Work out the finished part from the listing and answer in its coordinate system (mm). Face numbers are marked on the shaded views. A direction names the side the tool comes from. Coordinates: 2 decimals unless noted, no trailing zeros. Order: outer loops, then holes, each group sorted by start corner. A loop starts at its lowest first (then second) coordinate and runs counter-clockwise, first axis right, second up. Notation, with made-up numbers: (75, 31) - (129, 31) arc R10 ccw to (129, 43) - close; hole circle Ø8 at (31, 20.5). An arc over 180 degrees is marked (long way). Use CSV: the item, a comma, the result in double quotes. Start each with the question number.
from build123d import *

# Parameters (mm, degrees)
F0_W      = 18
F0_H      = 91.5
F0_W_2    = 7.2
F0_H_2    = 3.15
F0_W_3    = 12
F0_H_3    = 34
F1_DEPTH  = 10
F2_R      = 6
F4_DEPTH  = 7
F5_SIZE   = 2
F6_R      = 1.65
F7_DEPTH  = 25
F8_DEPTH  = 3
F10_R     = 4.99999
F12_DEPTH = 2.4
F15_DEPTH = 2.5
F17_R     = 2.15
F18_DEPTH = 20
F20_W     = 7.2
F20_H     = 3.15
F21_DEPTH = 1.25


# Not quite as in the source:
# - a fillet or chamfer is up to 0.001 mm smaller than in the source, because OpenCascade refuses the exact size


with BuildPart() as f1:
    # F0 (on Top) → F1 (new body)
    with BuildSketch(Plane.XY):
        with Locations((0.4665288143, 11.6095117688)):
            Rectangle(F0_W, F0_H)
        with Locations((0, -28.5654882312)):
            Rectangle(F0_W_2, F0_H_2, mode=Mode.SUBTRACT)
        Polygon((6.5, -24.9904882312), (-6.5, -24.9904882312), (-6.5, -15.9904882312), (0, -9.9904882312), (6.5, -15.9904882312), align=None, mode=Mode.SUBTRACT)
        with Locations((0.4665288143, 11.0095117688)):
            Rectangle(F0_W_3, F0_H_3, mode=Mode.SUBTRACT)
        with Locations((0.4665288143, 11.0095117688)):
            Rectangle(F0_W_3, F0_H_3)
    extrude(amount=F1_DEPTH)

    # F2
    f2_edges = [f1.edges().sort_by_distance(p)[0] for p in [
        (9.466529, -34.140488, 5),
        (-8.533471, -34.140488, 5),
    ]]
    fillet(f2_edges, radius=F2_R)

    # F0 (on Top) → F4 (cut)
    with BuildSketch(Plane.XY):
        with Locations((0.4665288143, 11.0095117688)):
            Rectangle(F0_W_3, F0_H_3)
    extrude(amount=F4_DEPTH, mode=Mode.SUBTRACT)

    # F5
    f5_edges = [f1.edges().sort_by_distance(p)[0] for p in [
        (6.466529, 11.009512, 7),
        (-5.533471, 11.009512, 7),
    ]]
    chamfer(f5_edges, length=F5_SIZE)

    # F6 (on offset) → F7 (cut)
    with BuildSketch(Plane.YZ.offset(9.4665288143)):
        with BuildLine():
            Line((40.3595117688, 3.35), (40.3595117688, 6.65))
            ThreePointArc((40.3595117688, 6.65), (38.7095117688, 5), (40.3595117688, 3.35))
        make_face()
        with BuildLine():
            ThreePointArc((42.0095117688, 5), (41.5262379578, 6.166726189), (40.3595117688, 6.65))
            Line((40.3595117688, 6.65), (40.3595117688, 3.35))
            ThreePointArc((40.3595117688, 3.35), (41.5262379578, 3.833273811), (42.0095117688, 5))
        make_face()
        with Locations((52.3595117688, 5)):
            Circle(F6_R)
    extrude(amount=-F7_DEPTH, mode=Mode.SUBTRACT)

    # F6 (on offset) → F8 (cut)
    with BuildSketch(Plane.YZ.offset(9.4665288143)):
        with BuildLine():
            Line((40.3595117688, 6.65), (40.3595117688, 7.9))
            ThreePointArc((40.3595117688, 7.9), (37.4595117688, 5), (40.3595117688, 2.1))
            Line((40.3595117688, 2.1), (40.3595117688, 3.35))
            ThreePointArc((40.3595117688, 3.35), (38.7095117688, 5), (40.3595117688, 6.65))
        make_face()
        with BuildLine():
            ThreePointArc((43.2595117688, 5), (42.4101214343, 7.0506096654), (40.3595117688, 7.9))
            Line((40.3595117688, 7.9), (40.3595117688, 6.65))
            ThreePointArc((40.3595117688, 6.65), (41.5262379578, 6.166726189), (42.0095117688, 5))
            ThreePointArc((42.0095117688, 5), (41.5262379578, 3.833273811), (40.3595117688, 3.35))
            Line((40.3595117688, 3.35), (40.3595117688, 2.1))
            ThreePointArc((40.3595117688, 2.1), (42.4101214343, 2.9493903346), (43.2595117688, 5))
        make_face()
    extrude(amount=-F8_DEPTH, mode=Mode.SUBTRACT)

    # F10 (radius 5 in the source; OpenCascade refuses exactly that, so slightly less here)
    f10_edges = [f1.edges().sort_by_distance(p)[0] for p in [
        (0.466529, 57.359512, 0),
        (0.466529, 57.359512, 10),
    ]]
    fillet(f10_edges, radius=F10_R)

    # F11 (on offset) → F12 (cut, symmetric)
    with BuildSketch(Plane.YZ):
        Polygon((47.8595117688, 0), (45.3595117688, 10), (35.3595117688, 10), (32.8595117688, 0), align=None)
    extrude(amount=F12_DEPTH, both=True, mode=Mode.SUBTRACT)

    # F14 (on offset) → F15 (cut)
    with BuildSketch(Plane(origin=(-8.5334711857, 0, 0), x_dir=(0, -1, 0), z_dir=(-1, 0, 0))):
        Polygon((-37.5882304767, 3.4), (-37.5882304767, 6.6), (-40.3595117688, 8.2), (-43.1307930609, 6.6), (-43.1307930609, 3.4), (-40.3595117688, 1.8), align=None)
    extrude(amount=-F15_DEPTH, mode=Mode.SUBTRACT)

    # F17 (on offset) → F18 (cut)
    with BuildSketch(Plane.XZ.offset(34.1404882312)):
        with Locations((0, 5)):
            Circle(F17_R)
    extrude(amount=-F18_DEPTH, mode=Mode.SUBTRACT)

    # F20 (on offset) → F21 (join)
    with BuildSketch(Plane.XY.offset(10)):
        with Locations((0, -28.5654882312)):
            Rectangle(F20_W, F20_H)
    extrude(amount=-F21_DEPTH)


solid = f1.part
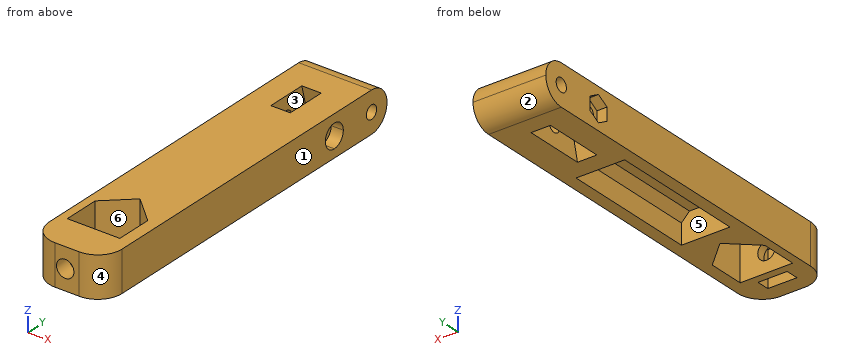
1) For a pull along X with two mould halves and no side action, classify the marked faces 1, 2 and 3 as +X half, -X half, draft (parallel to the pull), parting line (faces both ways), or undercut.
2) Flat-ended cylindrical pins translate along their axes: P1, Ø2, axis at x = -7, z = 5, coming from the -Y side; P2, Ø6.5, axis at x = 0, y = 7.5, coming from the -Z side. Find the tip coordinate at first contact, or state that the pin passes through.
3) For the marked faces 4, 5 and 6, determine the directions among +Z, -Z, +X, -X, +Y, -Y from which every point of the face is accessible in a straight line to the end or side of a thin tool.
4) Straight lines are drawn through the part: line 1 (Z direction, x = 0, y = -25.6); line 2 (Y direction, x = -3, z = 3.5); line 3 (Y direction, x = -3, z = 2). For each, find the intervals that lie inside material, in ascending order. Write a range as [from, to].
5) The part is cut by section A-A on y = 47. Determine the outline of the cut face in (x, z).
Answer key:
1,face 1,"+X half"
1,face 2,"draft"
1,face 3,"undercut"
2,P1,"y = -33.04"
2,P2,"z = 7"
3,face 4,"+Z, -Z, +X, -Y"
3,face 5,"-Z"
3,face 6,"+Z, -Z"
4,line 1,"[0, 2.85], [7.15, 10]"
4,line 2,"[-34.12, -30.14], [-26.99, -24.99], [-12.76, -5.99], [28.01, 39.67], [41.05, 51.67], [53.05, 57.13]"
4,line 3,"[-34.12, -30.14], [-26.99, -24.99], [-12.76, -5.99], [28.01, 56.36]"
5,outline,"(-8.53, 0) - (-2.4, 0) - (-2.4, 3.44) - (2.4, 3.44) - (2.4, 0) - (9.47, 0) - (9.47, 10) - (-8.53, 10) - close"
